For this review, take the finished solid that the model builds, in its own axes (mm). Coordinates: 2 decimals unless noted, no trailing zeros. Write each loop counter-clockwise with the first axis right and the second up, starting at its lowest first coordinate (ties: lowest second). Pieces come first, ordered by that corner, then holes. Notation, with made-up numbers: (29, 22.5) -> (70, 22.5) arc R10 cw to (70, 26.5) -> close; hole circle Ø6 at (42, 18.5). An arc over 180 degrees is marked (long way). One line per item, written item: value. Start each with the question number.
1) For probe 1 along X at (y, z) = (-4.5, -54); probe 2 along Z at (x, y) = (39.5, -4.5); probe 3 along X at (y, z) = (-6, -286), list the stretches that pass through material, from the lowest coordinate up. Write a range as from..to.
2) Add section A-A (x = -6). State the section outline as (y, z) points.
3) For pin 1 Ø5 at (y, z) = (-2.5, -111) entering from +X; pin 2 Ø10 at (x, z) = (56, -420) entering from +Y; pin 3 Ø4 at (y, z) = (-4.5, -178.5) entering from +X; pin 4 Ø4.5 at (x, y) = (-7.5, -5) entering from +Z, all flat-tipped, find the tip position at first contact; note any pin that passes through.
from build123d import *

# Parameters (mm, degrees)
F1_DEPTH = 8.89


with BuildPart() as f1:
    # F0 (on Front) → F1 (new body)
    with BuildSketch(Plane.XZ):
        with BuildLine():
            Line((152.4, 0), (127, 0))
            add(Edge.make_bspline(
                [(127, 0), (127, -20.0168341398), (123.3922770096, -58.2410161724), (89.3160713506, -123.1038827606), (57.5735042432, -125.7764468865), (43.5800775886, -127)],
                knots=[0, 0, 0, 0, 0.345812323, 0.7105558481, 1, 1, 1, 1], degree=3))
            Line((43.5800775886, -127), (0, -127))
            Line((0, -127), (-43.5800775886, -127))
            add(Edge.make_bspline(
                [(-127, 0), (-127, -20.0168341398), (-123.3922770096, -58.2410161724), (-89.3160713506, -123.1038827606), (-57.5735042432, -125.7764468865), (-43.5800775886, -127)],
                knots=[0, 0, 0, 0, 0.345812323, 0.7105558481, 1, 1, 1, 1], degree=3))
            Line((-127, 0), (-152.4, 0))
            add(Edge.make_bspline(
                [(-152.4, 0), (-150.2703878505, -31.3639571024), (-146.3939702155, -88.3715453558), (-110.9714635835, -160.9462971944), (-158.6767490389, -174.9726116512), (-154.2449504284, -190.6305366091), (-152.4, -197.1800625324)],
                knots=[0, 0, 0, 0, 0.3476574396, 0.6384459753, 0.8455987873, 1, 1, 1, 1], degree=3))
            add(Edge.make_bspline(
                [(-152.4, -197.1800625324), (-148.2010351465, -226.5358633988), (-138.5263708492, -292.0003756963), (-159.3646682678, -437.8166234112), (-168.1102758726, -487.6635444085), (-172.8998571634, -508)],
                knots=[0, 0, 0, 0, 0.3238760373, 0.7228207872, 1, 1, 1, 1], degree=3))
            Line((-172.8998571634, -508), (0, -508))
            Line((0, -508), (172.8998571634, -508))
            add(Edge.make_bspline(
                [(152.4, -197.1800625324), (148.2010351465, -226.5358633988), (138.5263708492, -292.0003756963), (159.3646682678, -437.8166234112), (168.1102758726, -487.6635444085), (172.8998571634, -508)],
                knots=[0, 0, 0, 0, 0.3238760373, 0.7228207872, 1, 1, 1, 1], degree=3))
            add(Edge.make_bspline(
                [(152.4, 0), (150.2703878505, -31.3639571024), (146.3939702155, -88.3715453558), (110.9714635835, -160.9462971944), (158.6767490389, -174.9726116512), (154.2449504284, -190.6305366091), (152.4, -197.1800625324)],
                knots=[0, 0, 0, 0, 0.3476574396, 0.6384459753, 0.8455987873, 1, 1, 1, 1], degree=3))
        make_face()
    extrude(amount=F1_DEPTH)


solid = f1.part
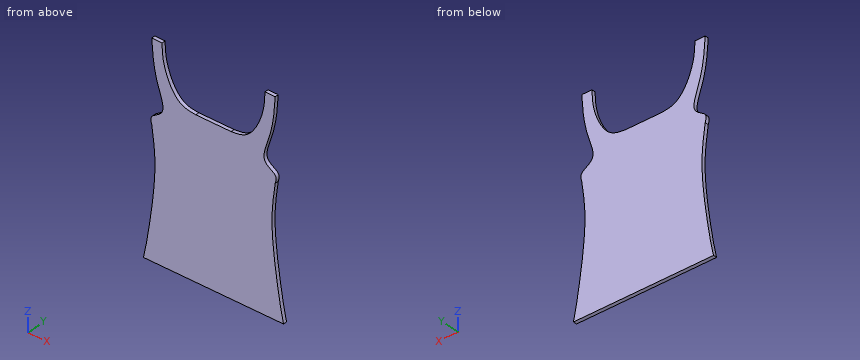
Numbers:
1. probe 1: -147.41..-120.17, 120.17..147.41
1. probe 2: -508..-127
1. probe 3: -144.44..144.44
2. outline: (-8.89, -508) -> (0, -508) -> (0, -127) -> (-8.89, -127) -> close
3. pin 1: x = 134.23
3. pin 2: y = 0
3. pin 3: x = 153.45
3. pin 4: z = -127
